Check sheet for the modelled part. Datum: model origin and axes. Units: mm. A direction names the side the tool comes from. Coordinates: 2 decimals unless noted, no trailing zeros. Write each loop counter-clockwise with the first axis right and the second up, starting at its lowest first coordinate (ties: lowest second). Pieces come first, ordered by that corner, then holes. Notation, with made-up numbers: (43.5, 55) -> (90.5, 55) arc R27 cw to (90.5, 75) -> close; hole circle Ø1 at (-38, 49). An arc over 180 degrees is marked (long way). One line per item, written item: value. Start each with the question number.
1) Sectioned sample at C-C on z = -13. Enter the section's corners in (x, y).
2) Draft check along X on faces 4 (the cylindrical face through (-10.173, -14.95, 34.286)), 5 (the flat face through (34.7, -2.46, -15.13)), 6 (the flat face through (-13.45, -97.54, -62.17)). Enter one of: +X half, -X half, draft (parallel to the pull), parting line (faces both ways), or undercut.
3) Sectioned sample at B-B on y = -35. Enter the section's corners in (x, z), plus the area to 3 significant figures.
4) Scan lines: line 1 along Y through (x, z) = (-22, 25); line 2 along X through (y, z) = (-21, 24.5); line 3 along X through (y, z) = (-57.5, 28). Record each from-to range of solid material in increasing order. Write a range as [from, to].
5) Sectioned sample at A-A on z = 26.5. Enter the section's corners in (x, y).
6) Gauge pin test, flat ends, axial feed: P1, Ø22, axis at x = -10.5, y = -112.5, coming from the -Z side; P2, Ø10, axis at y = -112.5, z = -20, coming from the +X side; P3, Ø7.5, axis at x = -3.5, z = 25, coming from the -Y side. Record the tip position at first contact, or that the pin passes through.
7) Set-up check for faces 1 (the flat face through (-11, -83.605, 23)), 2 (the flat face through (-11, -110, -45.558)), 3 (the flat face through (-11, -110, 16.076)): record each of +Z, -Z, +X, -X, +Y, -Y from which the full face is reachable in a straight line by a thin tool's end or side.
8) Sectioned sample at D-D on x = -51.5. Enter the section's corners in (y, z).
```python
from build123d import *

# Parameters (mm, degrees)
F0_W     = 100.1162827015
F0_H     = 100.4215180874
F1_DEPTH = 100
F2_SIZE  = 5
F3_W     = 68.8809547573
F3_H     = 61.6337545216
F4_DEPTH = 25
F5_R     = 5
F6_W     = 68.3720968664
F6_H     = 67.151170224
F7_DEPTH = 25
F8_R     = 5


with BuildPart() as f1:
    # F0 (on Front) → F1 (new body)
    with BuildSketch(Plane.XZ):
        with Locations((-12.8197669983, -14.4985467196)):
            Rectangle(F0_W, F0_H)
    extrude(amount=F1_DEPTH)

    # F2
    f2_edges = [f1.edges().sort_by_distance(p)[0] for p in [
        (37.238374, -50, -64.709306),
        (-62.877908, -50, 35.712212),
        (-12.819767, -100, 35.712212),
        (-12.819767, 0, 35.712212),
        (37.238374, -50, 35.712212),
        (-12.819767, -100, -64.709306),
        (-12.819767, 0, -64.709306),
        (-62.877908, -100, -14.498547),
        (-62.877908, -50, -64.709306),
        (37.238374, -100, -14.498547),
        (-62.877908, 0, -14.498547),
        (37.238374, 0, -14.498547),
    ]]
    chamfer(f2_edges, length=F2_SIZE)

    # F3 (on face) → F4 (join)
    with BuildSketch(Plane.XZ.offset(100)):
        with Locations((-10.0983185694, -14.7410277277)):
            Rectangle(F3_W, F3_H)
    extrude(amount=F4_DEPTH)

    # F5
    f5_edges = [f1.edges().sort_by_distance(p)[0] for p in [
        (-10.098319, -125, 16.07585),
        (24.342159, -125, -14.741028),
        (24.342159, -112.5, 16.07585),
        (24.342159, -112.5, -45.557905),
        (-10.098319, -125, -45.557905),
        (-44.538796, -112.5, -45.557905),
        (-44.538796, -125, -14.741028),
        (-44.538796, -112.5, 16.07585),
    ]]
    fillet(f5_edges, radius=F5_R)

    # F6 (on face) → F7 (cut)
    with BuildSketch(Plane.XY.offset(35.7122123241)):
        with Locations((-10.5813946575, -50.0290710479)):
            Rectangle(F6_W, F6_H)
    extrude(amount=-F7_DEPTH, mode=Mode.SUBTRACT)

    # F8
    f8_edges = [f1.edges().sort_by_distance(p)[0] for p in [
        (-10.581395, -16.453486, 10.712212),
        (-44.767443, -50.029071, 10.712212),
        (-10.581395, -83.604656, 10.712212),
        (23.604654, -50.029071, 10.712212),
        (23.604654, -16.453486, 23.212212),
        (-44.767443, -16.453486, 23.212212),
        (-44.767443, -83.604656, 23.212212),
        (-44.767443, -50.029071, 35.712212),
        (23.604654, -83.604656, 23.212212),
        (23.604654, -50.029071, 35.712212),
        (-10.581395, -83.604656, 35.712212),
        (-10.581395, -16.453486, 35.712212),
    ]]
    fillet(f8_edges, radius=F8_R)


solid = f1.part
```
Answers:
1. outline: (-62.88, -95) -> (-57.88, -100) -> (-44.54, -100) -> (-44.54, -120) arc R5 ccw to (-39.54, -125) -> (19.34, -125) arc R5 ccw to (24.34, -120) -> (24.34, -100) -> (32.24, -100) -> (37.24, -95) -> (37.24, -5) -> (32.24, 0) -> (-57.88, 0) -> (-62.88, -5) -> close
2. face 4: undercut
2. face 5: +X half
2. face 6: draft
3. outline: (-62.88, -59.71) -> (-57.88, -64.71) -> (32.24, -64.71) -> (37.24, -59.71) -> (37.24, 30.71) -> (32.24, 35.71) -> (28.6, 35.71) arc R5 ccw to (23.6, 30.71) -> (23.6, 15.71) arc R5 cw to (18.6, 10.71) -> (-39.77, 10.71) arc R5 cw to (-44.77, 15.71) -> (-44.77, 30.71) arc R5 ccw to (-49.77, 35.71) -> (-57.88, 35.71) -> (-62.88, 30.71) -> close
3. area: 8,290 mm2
4. line 1: y = [-100, -83.6], [-16.45, 0]
4. line 2: x = [-62.88, -44.75], [23.58, 37.24]
4. line 3: x = [-62.88, -44.77], [23.6, 37.24]
5. outline: (-62.88, -95) -> (-57.88, -100) -> (32.24, -100) -> (37.24, -95) -> (37.24, -5) -> (32.24, 0) -> (-57.88, 0) -> (-62.88, -5) -> close; hole (-44.77, -78.6) arc R5 ccw to (-39.77, -83.6) -> (18.6, -83.6) arc R5 ccw to (23.6, -78.6) -> (23.6, -21.45) arc R5 ccw to (18.6, -16.45) -> (-39.77, -16.45) arc R5 ccw to (-44.77, -21.45) -> close
6. P1: stops at z = -45.56
6. P2: stops at x = 24.34
6. P3: stops at y = -100
7. face 1: +Z
7. face 2: -Z, +X, -X, -Y
7. face 3: +Z, +X, -X, -Y
8. outline: (-100, -59.71) -> (-95, -64.71) -> (-5, -64.71) -> (0, -59.71) -> (0, 30.71) -> (-5, 35.71) -> (-95, 35.71) -> (-100, 30.71) -> close
